Geometry check sheet. Reference: the model listing, model coordinates, mm. Face numbers are marked on the shaded views. A direction names the side the tool comes from. Coordinates: 2 decimals unless noted, no trailing zeros. Write each loop counter-clockwise with the first axis right and the second up, starting at its lowest first coordinate (ties: lowest second). Pieces come first, ordered by that corner, then holes. Notation, with made-up numbers: (30.25, 3) -> (35.25, 3) arc R4 cw to (35.25, 9) -> close; hole circle Ø7 at (65, 9.25). An arc over 180 degrees is marked (long way). Use a Markdown table: item, result.
```python
from build123d import *

# Parameters (mm, degrees)
F0_W        = 165
F0_H        = 80
F0_W_2      = 151.5524461865
F0_H_2      = 1.4
F0_W_3      = 1.4
F0_H_3      = 76.4191485941
F0_H_4      = 76.5563435853
F0_W_4      = 151.9825384021
F0_H_5      = 54.7616053373
F0_W_5      = 152.1170958877
F1_DEPTH    = 21.11
F2_T1_DEPTH = 265
F3_DEPTH    = 8
F4_R        = 5


# Not quite as in the source:
# - a fillet or chamfer that OpenCascade refuses, or shapes differently, is made with other operations: its cross-section is extruded or revolved along the edge and cut away or added


with BuildPart() as f1:
    # F0 (on Top) → F1 (new body)
    with BuildSketch(Plane.XY):
        with Locations((-0.5210009217, 2.8526327014)):
            Rectangle(F0_W, F0_H)
        with Locations((-0.6515718997, -33.7715006649)):
            Rectangle(F0_W_2, F0_H_2, mode=Mode.SUBTRACT)
        with Locations((-80.7459980965, 2.6404876262)):
            Rectangle(F0_W_3, F0_H_3, mode=Mode.SUBTRACT)
        with Locations((79.2265801907, 2.7090851218)):
            Rectangle(F0_W_3, F0_H_4, mode=Mode.SUBTRACT)
        with Locations((-0.4365257919, 8.6810430512)):
            Rectangle(F0_W_4, F0_H_5, mode=Mode.SUBTRACT)
        with Locations((-0.4392154515, 40.7097370148)):
            Rectangle(F0_W_5, F0_H_2, mode=Mode.SUBTRACT)
    extrude(amount=F1_DEPTH)

    # F2: fillet of radius 20 on 1 edges, made by hand

    # F2_s2 → F2_t1 (cut)
    with BuildSketch(Plane.YZ.offset(-133.0210009217)):
        with BuildLine():
            ThreePointArc((-37.1473672986, 1.11), (-31.2895029223, 15.2521356237), (-17.1473672986, 21.11))
            Line((-17.1473672986, 21.11), (-37.1473672986, 21.11))
            Line((-37.1473672986, 21.11), (-37.1473672986, 1.11))
        make_face()
    extrude(amount=F2_T1_DEPTH, mode=Mode.SUBTRACT)

    # F0 (on Top) → F3 (join)
    with BuildSketch(Plane.XY):
        with Locations((-0.4365257919, 8.6810430512)):
            Rectangle(F0_W_4, F0_H_5)
    extrude(amount=F3_DEPTH)

    # F4
    f4_edges = [f1.edges().sort_by_distance(p)[0] for p in [
        (-83.021001, 42.852633, 10.555),
        (81.978999, 42.852633, 10.555),
    ]]
    fillet(f4_edges, radius=F4_R)


solid = f1.part
```
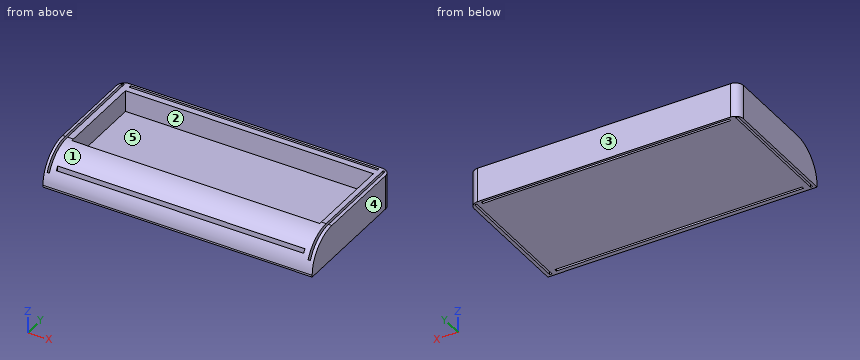
Item 1: Section check D-D on z = 5.75. Record the boundary of the cut face in (x, y), then the cut area to 3 significant figures.
Answer block:
| item | result |
|---|---|
| outline | (-83.02, -36.6) -> (81.98, -36.6) -> (81.98, 37.85) arc R5 ccw to (76.98, 42.85) -> (-78.02, 42.85) arc R5 ccw to (-83.02, 37.85) -> close; hole (-81.45, -35.57) -> (-80.05, -35.57) -> (-80.05, 40.85) -> (-81.45, 40.85) -> close; hole (-76.5, 40.01) -> (75.62, 40.01) -> (75.62, 41.41) -> (-76.5, 41.41) -> close; hole (-76.43, -34.47) -> (75.12, -34.47) -> (75.12, -33.07) -> (-76.43, -33.07) -> close; hole (78.53, -35.57) -> (79.93, -35.57) -> (79.93, 40.99) -> (78.53, 40.99) -> close |
| area | 12,500 mm^2 |
Item 2: Section check B-B on y = 4.5. Record the boundary of the cut face in (x, z).
Answer block:
| item | result |
|---|---|
| outline | (-83.02, 0) -> (-81.45, 0) -> (-81.45, 21.11) -> (-83.02, 21.11) -> close; (-80.05, 0) -> (78.53, 0) -> (78.53, 21.11) -> (75.55, 21.11) -> (75.55, 8) -> (-76.43, 8) -> (-76.43, 21.11) -> (-80.05, 21.11) -> close; (79.93, 0) -> (81.98, 0) -> (81.98, 21.11) -> (79.93, 21.11) -> close |
Item 3: Section check A-A on x = -21.5. Record the boundary of the cut face in (y, z), then the cut area to 3 significant figures.
Answer block:
| item | result |
|---|---|
| outline | (-37.15, 0) -> (-34.47, 0) -> (-34.47, 11.1) arc R20 ccw to (-37.15, 1.11) -> close; (-33.07, 0) -> (40.01, 0) -> (40.01, 21.11) -> (36.06, 21.11) -> (36.06, 8) -> (-18.7, 8) -> (-18.7, 21.05) arc R20 ccw to (-33.07, 13.21) -> close; (41.41, 0) -> (42.85, 0) -> (42.85, 21.11) -> (41.41, 21.11) -> close |
| area | 838 mm^2 |
Item 4: Section check C-C on z = 15.25. Record the boundary of the cut face in (x, y), then the cut area to 3 significant figures.
Answer block:
| item | result |
|---|---|
| outline | (-83.02, -31.29) -> (-81.45, -31.29) -> (-81.45, 40.85) -> (-80.05, 40.85) -> (-80.05, -31.29) -> (78.53, -31.29) -> (78.53, 40.99) -> (79.93, 40.99) -> (79.93, -31.29) -> (81.98, -31.29) -> (81.98, 37.85) arc R5 ccw to (76.98, 42.85) -> (-78.02, 42.85) arc R5 ccw to (-83.02, 37.85) -> close; hole (-76.5, 40.01) -> (75.62, 40.01) -> (75.62, 41.41) -> (-76.5, 41.41) -> close; hole (-76.43, -18.7) -> (75.55, -18.7) -> (75.55, 36.06) -> (-76.43, 36.06) -> close |
| area | 3,490 mm^2 |
Item 5: Mould release check, pull along X, two halves, no side actions. Record for the marked faces 3, 4 and 5: +X half, -X half, draft (parallel to the pull), parting line (faces both ways), or undercut.
Answer block:
| item | result |
|---|---|
| face 3 | draft |
| face 4 | +X half |
| face 5 | undercut |
Item 6: Depth check by flat-ended pin: P1, Ø5, axis at x = -14.5, z = 5, coming from the -Y side; P2, Ø0.7, axis at x = 79.5, z = 15.5, coming from the -Y side; P3, Ø1.1, axis at y = 40.5, z = 14.5, coming from the +X side. Enter the tip coordinate at first touch or a pass-through.
Answer block:
| item | result |
|---|---|
| P1 | stops at y = -37.1 |
| P2 | stops at y = 40.99 |
| P3 | stops at x = 81.52 |
Item 7: Tool access check on the marked faces 1 and 2. Record the directions out of +Z, -Z, +X, -X, +Y, -Y that give a thin tool (end or side, any length) a straight path to the whole face; none if there is none.
Answer block:
| item | result |
|---|---|
| face 1 | +Z, +X, -X, -Y |
| face 2 | +Z |
Item 8: Thickness scan on L1, parallel to X at y = 37, z = 9.75; L2, parallel to X at y = -12.5, z = 17.5; L3, parallel to Y at x = -35.5, z = 1.25. Record the ranges inside material, lowest first. Write a range as [from, to].
Answer block:
| item | result |
|---|---|
| L1 | x = [-83.02, -81.45], [-80.05, 78.53], [79.93, 81.98] |
| L2 | x = [-83.02, -81.45], [-80.05, -76.43], [75.55, 78.53], [79.93, 81.98] |
| L3 | y = [-37.15, -34.47], [-33.07, 40.01], [41.41, 42.85] |
